The drawing under review shows one solid part. Ordinate dimensions are in mm from its lowest x, y, z. A direction names the side the tool comes from. Coordinates: 2 decimals unless noted, no trailing zeros. Loops run counter-clockwise (first coordinate to the right, second up) from the corner with the lowest first, then second, coordinate; pieces in that order, holes last. Notation, with made-up numbers: M 13.25,-34.5 L 63.25,-34.5 A36 cw 63.25,3.5 Z; hole C 26.5,73.5 d3. An arc over 180 degrees is marked long. Answer as CSV lines item,"result". Start each with the question number.
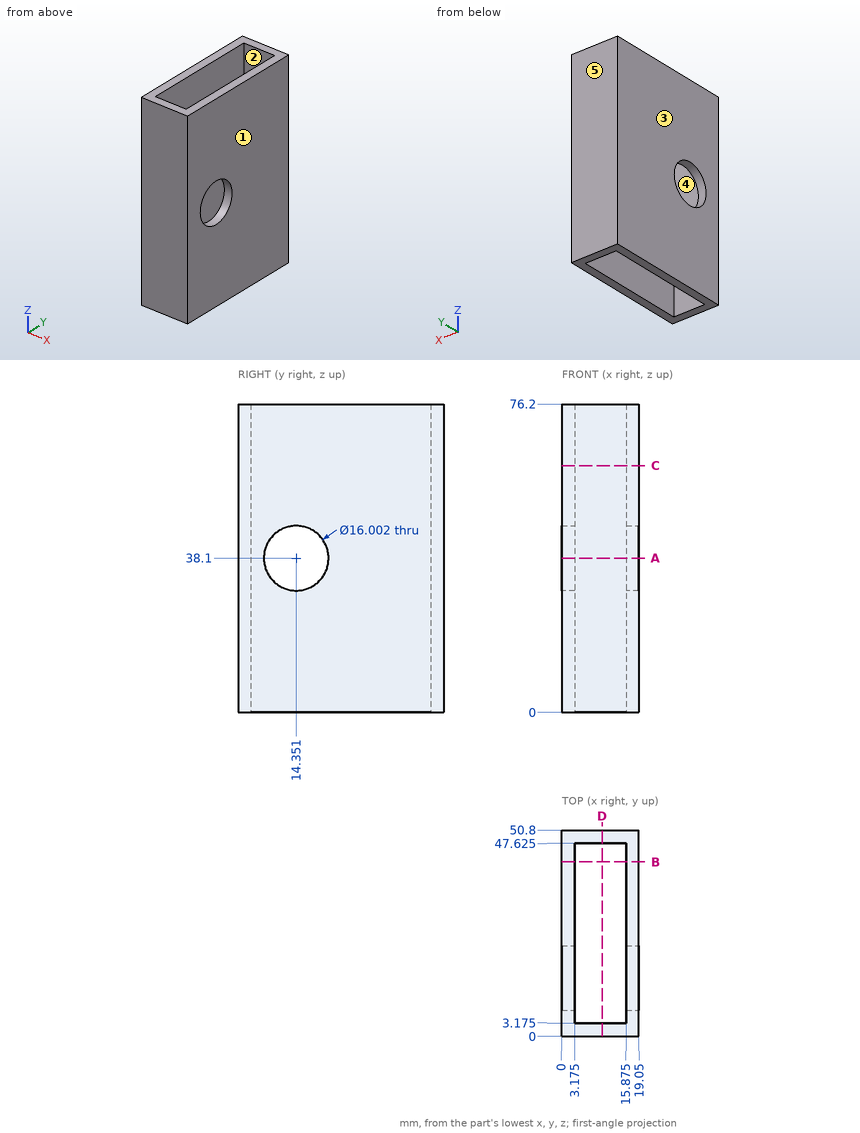
Item 1: Add section C-C (z = 61). Give the boundary of the cut face in (x, y) (3 decimals), plus the area to 3 significant figures.
Item 2: For pin 1 (5 mm diameter, centred on x = 6, z = 56, fed in from -Y), flat-tipped, find the tip position at first contact; note if it passes through.
Item 3: Add section B-B (y = 43). Give the boundary of the cut face in (x, z) (3 decimals).
Item 4: Add section A-A (z = 38.1). Give the boundary of the cut face in (x, y) (3 decimals).
Item 5: Mouldability with a two-part tool opening along X and no side actions: class the marked faces 3, 4 and 5 as released by +X, released by -X, zero draft, split by the parting line, or undercut.
Item 6: Add section D-D (x = 10). Give the boundary of the cut face in (y, z) (3 decimals).
Item 7: For line 1 along X through (y, z) = (24, 29.5) (3 decimals); line 2 along Y through (x, z) = (6, 53.5) (3 decimals); line 3 along Y through (x, z) = (17.8, 38.1), list the stretches that pass through material, from the lowest coordinate up. Write a range as from..to.
Item 8: For the marked faces 1 and 2, list the 3-axis set-ups (+Z, -Z, +X, -X, +Y, -Y) from which the entire face can be reached by the end or side of a thin tool; tool diameter is ignored.
Response:
1,outline,"M 0,0 L 19.05,0 L 19.05,50.8 L 0,50.8 Z; hole M 3.175,3.175 L 15.875,3.175 L 15.875,47.625 L 3.175,47.625 Z"
1,area,"403 mm²"
2,pin 1,"y = 0"
3,outline,"M 0,0 L 3.175,0 L 3.175,76.2 L 0,76.2 Z; M 15.875,0 L 19.05,0 L 19.05,76.2 L 15.875,76.2 Z"
4,outline,"M 0,0 L 19.05,0 L 19.05,6.35 L 15.875,6.35 L 15.875,3.175 L 3.175,3.175 L 3.175,6.35 L 0,6.35 Z; M 0,22.352 L 3.175,22.352 L 3.175,47.625 L 15.875,47.625 L 15.875,22.352 L 19.05,22.352 L 19.05,50.8 L 0,50.8 Z"
5,face 3,"released by -X"
5,face 4,"undercut"
5,face 5,"zero draft"
6,outline,"M 0,0 L 3.175,0 L 3.175,76.2 L 0,76.2 Z; M 47.625,0 L 50.8,0 L 50.8,76.2 L 47.625,76.2 Z"
7,line 1,"0..3.175, 15.875..19.05"
7,line 2,"0..3.175, 47.625..50.8"
7,line 3,"0..6.35, 22.35..50.8"
8,face 1,"+Z, -Z, +X, +Y, -Y"
8,face 2,"+Z, -Z"
